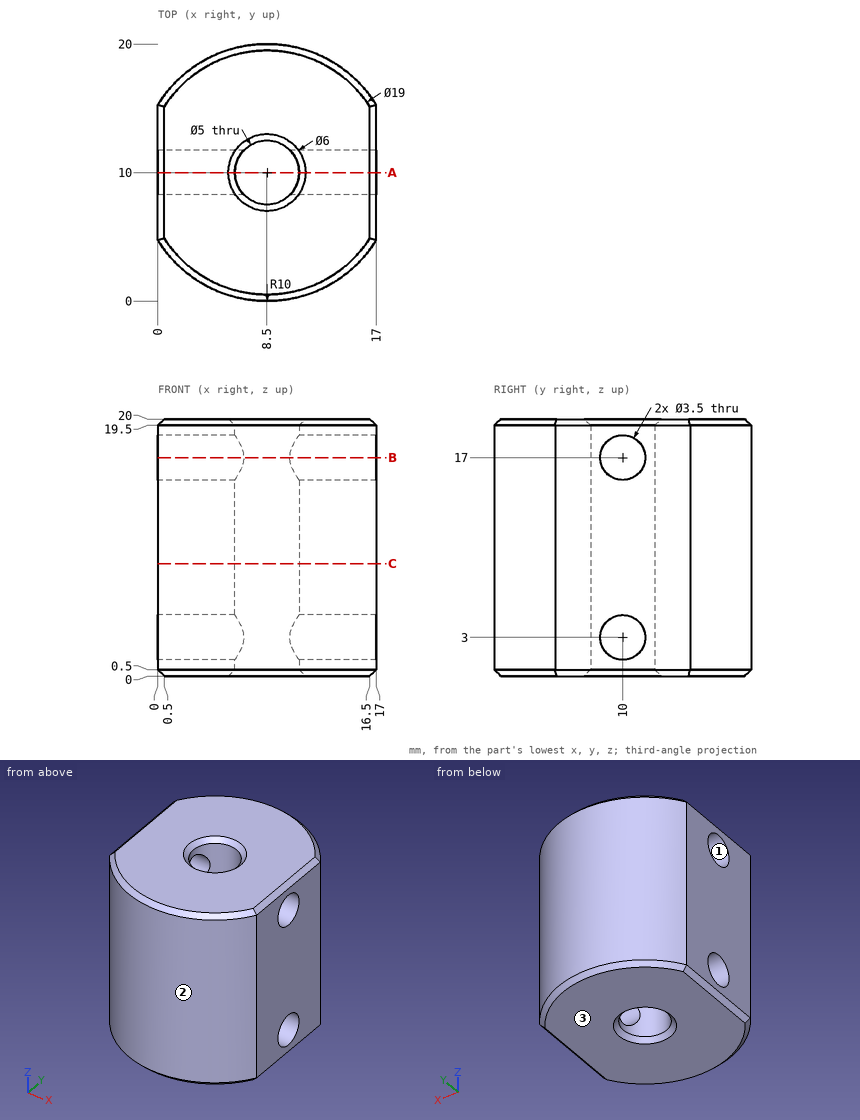
Could you check a few things on this drawing? It's one solid part, dimensions in mm from its lowest x, y, z. Coordinates: 2 decimals unless noted, no trailing zeros. Order: outer loops, then holes, each group sorted by start corner. A loop starts at its lowest first (then second) coordinate and runs counter-clockwise, first axis right, second up. Notation, with made-up numbers: M 22,87.5 L 72,87.5 A24 ccw 72,101.5 Z; hole C -19.75,74.5 d2. An arc over 180 degrees is marked long. Use a Markdown table: item, result. Add a question column.
Q1. If I drill on L1, parallel to Z at x = 13.25, y = 10; L2, parallel to X at y = 10, z = 12.5; L3, parallel to Z at x = 3, y = 9.25, over which ranges is the centre line in solid material (lowest first)?
Q2. I want a section at C-C on z = 8.75. List the corners of the cut face in (x, y) for me, then the cut area to 3 significant figures.
Q3. I want a section at B-B on z = 17. List the corners of the cut face in (x, y) for me, then the cut area to 3 significant figures.
Q4. I'm going to push a flat-ended pin straight in: pin 1 (1 mm diameter, centred on x = 6.5, z = 8, fed in from +Y). Where does the tip first touch, or does it pass through?
Q5. We'd pull the mould along Y, two halves only. Please class the marked faces 1, 2 and 3: pulls with the +Y half, pulls with the -Y half, needs draft (parallel to the pull), parting line crosses it, or undercut.
Q6. I want a section at A-A on y = 10. Give the number of separate pieces and of enclosed holes in the cut face, then the cut area to 3 significant figures.
Checked values:
| question | item | result |
|---|---|---|
| 1 | L1 | 0 to 1.25, 4.75 to 15.25, 18.75 to 20 |
| 1 | L2 | 0 to 6, 11 to 17 |
| 1 | L3 | 0 to 1.42, 4.58 to 15.42, 18.58 to 20 |
| 2 | outline | M 0,4.73 A10 ccw 17,4.73 L 17,15.27 A10 ccw 0,15.27 Z; hole C 8.5,10 d5 |
| 2 | area | 273 mm² |
| 3 | outline | M 0,4.73 A10 ccw 17,4.73 L 17,8.25 L 10.29,8.25 A2.5 cw 6.71,8.25 L 0,8.25 Z; M 0,11.75 L 6.71,11.75 A2.5 cw 10.29,11.75 L 17,11.75 L 17,15.27 A10 ccw 0,15.27 Z |
| 3 | area | 230 mm² |
| 4 | pin 1 | y = 19.89 |
| 5 | face 1 | undercut |
| 5 | face 2 | pulls with the -Y half |
| 5 | face 3 | needs draft |
| 6 | separate pieces | 6 |
| 6 | enclosed holes | 0 |
| 6 | area | 155 mm² |
